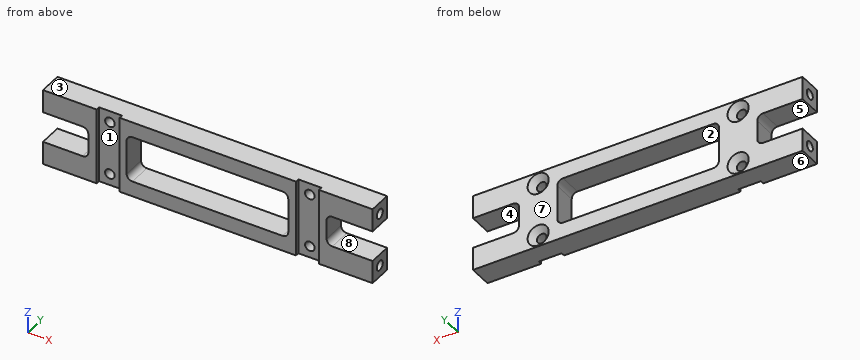
```python
from build123d import *

# Parameters (mm, degrees)
SKETCH2_W                   = 86
SKETCH2_H                   = 20
BOSS_EXTRUDE1_DEPTH         = 6
TAP_DRILL_FOR_M3_TAP2_D     = 2.5
TAP_DRILL_FOR_M3_TAP2_DEPTH = 8
TAP_DRILL_FOR_M3_TAP2_TIP   = 0.751075774
TAP_DRILL_FOR_M3_TAP1_D     = 2.5
TAP_DRILL_FOR_M3_TAP1_DEPTH = 8
TAP_DRILL_FOR_M3_TAP1_TIP   = 0.751075774
SKETCH7_W                   = 6
SKETCH7_H                   = 20
CUT_EXTRUDE1_DEPTH          = 1
TAP_DRILL_FOR_M3X0_5_TAP1_D = 2.5
CHAMFER1_SIZE               = 1.5
CUT_EXTRUDE2_REACH          = 90.499
SKETCH9_W                   = 42.171572875
SKETCH9_H                   = 12
SKETCH9_W_2                 = 11.828427125
SKETCH9_H_2                 = 8
SKETCH9_W_3                 = 12
FILLET1_R                   = 1.5


with BuildPart() as part:
    # Sketch2 → Boss-Extrude1 (new body)
    with BuildSketch(Plane(origin=(0, 0, 0), x_dir=(1, 0, 0), z_dir=(0, 1, 0))):
        with Locations((43, -10)):
            Rectangle(SKETCH2_W, SKETCH2_H)
    extrude(amount=BOSS_EXTRUDE1_DEPTH)

    # Tap Drill for M3 Tap2
    with Locations(Plane(origin=(86, 0.779165189, 7.640466368), x_dir=(0, 0, -1), z_dir=(1, 0, 0))):
        with Locations((-9.359533632, 2.220834811), (4.640466368, 2.220834811)):
            Hole(TAP_DRILL_FOR_M3_TAP2_D / 2, depth=TAP_DRILL_FOR_M3_TAP2_DEPTH)
            with Locations((0, 0, -(TAP_DRILL_FOR_M3_TAP2_DEPTH + TAP_DRILL_FOR_M3_TAP2_TIP / 2))):  # 118° drill point
                Cone(0, TAP_DRILL_FOR_M3_TAP2_D / 2, TAP_DRILL_FOR_M3_TAP2_TIP, mode=Mode.SUBTRACT)

    # Tap Drill for M3 Tap1
    with Locations(Plane.ZY):
        with Locations((3, 3), (17, 3)):
            Hole(TAP_DRILL_FOR_M3_TAP1_D / 2, depth=TAP_DRILL_FOR_M3_TAP1_DEPTH)
            with Locations((0, 0, -(TAP_DRILL_FOR_M3_TAP1_DEPTH + TAP_DRILL_FOR_M3_TAP1_TIP / 2))):  # 118° drill point
                Cone(0, TAP_DRILL_FOR_M3_TAP1_D / 2, TAP_DRILL_FOR_M3_TAP1_TIP, mode=Mode.SUBTRACT)

    # Sketch7 → Cut-Extrude1 (cut)
    with BuildSketch(Plane.XZ):
        with Locations((17, 10)):
            Rectangle(SKETCH7_W, SKETCH7_H)
        with Locations((69, 10)):
            Rectangle(SKETCH7_W, SKETCH7_H)
    extrude(amount=-CUT_EXTRUDE1_DEPTH, mode=Mode.SUBTRACT)

    # Tap Drill for M3x0.5 Tap1 (through all)
    with Locations(Plane(origin=(16.828427125, 1, 17), x_dir=(0, 0, -1), z_dir=(0, -1, 0))):
        with Locations((0, 0), (14, 0), (0, 52.171572875), (14, 52.171572875)):
            Hole(TAP_DRILL_FOR_M3X0_5_TAP1_D / 2)

    # Chamfer1
    chamfer1_edges = [part.edges().sort_by_distance(p)[0] for p in [
        (69, 6, 1.75),
        (69, 6, 15.75),
        (16.828427125, 6, 1.75),
        (16.828427125, 6, 15.75),
    ]]
    chamfer(chamfer1_edges, length=CHAMFER1_SIZE)

    # Sketch9 → Cut-Extrude2 (cut, up to next)
    with BuildSketch(Plane(origin=(0, 6, 0), x_dir=(1, 0, 0), z_dir=(0, 1, 0)), mode=Mode.PRIVATE) as cut_extrude2_sk1:
        with Locations((42.914213563, -10)):
            Rectangle(SKETCH9_W, SKETCH9_H)
    cut_extrude2_tool1 = extrude(cut_extrude2_sk1.sketch, amount=-CUT_EXTRUDE2_REACH, mode=Mode.PRIVATE) & part.part
    # Sketch9 → Cut-Extrude2 (cut, up to next)
    with BuildSketch(Plane(origin=(0, 6, 0), x_dir=(1, 0, 0), z_dir=(0, 1, 0)), mode=Mode.PRIVATE) as cut_extrude2_sk2:
        with Locations((5.914213563, -10)):
            Rectangle(SKETCH9_W_2, SKETCH9_H_2)
    cut_extrude2_tool2 = extrude(cut_extrude2_sk2.sketch, amount=-CUT_EXTRUDE2_REACH, mode=Mode.PRIVATE) & part.part
    # Sketch9 → Cut-Extrude2 (cut, up to next)
    with BuildSketch(Plane(origin=(0, 6, 0), x_dir=(1, 0, 0), z_dir=(0, 1, 0)), mode=Mode.PRIVATE) as cut_extrude2_sk3:
        with Locations((80, -10)):
            Rectangle(SKETCH9_W_3, SKETCH9_H_2)
    cut_extrude2_tool3 = extrude(cut_extrude2_sk3.sketch, amount=-CUT_EXTRUDE2_REACH, mode=Mode.PRIVATE) & part.part
    add(cut_extrude2_tool1.solids().sort_by_distance((42.914214, 6, 10))[0], mode=Mode.SUBTRACT)
    add(cut_extrude2_tool2.solids().sort_by_distance((5.914214, 6, 10))[0], mode=Mode.SUBTRACT)
    add(cut_extrude2_tool3.solids().sort_by_distance((80, 6, 10))[0], mode=Mode.SUBTRACT)

    # Fillet1
    fillet1_edges = [part.edges().sort_by_distance(p)[0] for p in [
        (21.828427125, 3, 16),
        (21.828427125, 3, 4),
        (64, 3, 4),
        (64, 3, 16),
        (11.828427125, 3, 6),
        (11.828427125, 3, 14),
        (74, 3, 14),
        (74, 3, 6),
    ]]
    fillet(fillet1_edges, radius=FILLET1_R)


solid = part.part
```
Can you work these out from the model? Positions are in its coordinate system, mm. Face numbers are marked on the shaded views. A direction names the side the tool comes from. Coordinates: 2 decimals unless noted, no trailing zeros. Write each loop counter-clockwise with the first axis right and the second up, starting at its lowest first coordinate (ties: lowest second). Pieces come first, ordered by that corner, then holes. Notation, with made-up numbers: (48, -33) - (86, -33) arc R22 cw to (86, -2) - close; hole circle Ø7 at (55, 4). An arc over 180 degrees is marked (long way). Return JSON: item names as keys, results as strings.
Q1. I'm going to push flat-ended pins straight in: pin 1 Ø2 at (y, z) = (3, 3) entering from -X; pin 2 Ø1.1 at (y, z) = (0.5, 10.5) entering from -X; pin 3 Ø3 at (x, z) = (70, 12) entering from -Y; pin 4 Ø6.5 at (x, z) = (15.5, 10) entering from -Y. Where does each tip first touch, or does it pass through?
Computed values:
{"pin 1": "stops at x = 8.15", "pin 2": "stops at x = 11.83", "pin 3": "stops at y = 1", "pin 4": "stops at y = 0"}
Q2. If we section it at A-A (x = 58): Please give me the cut outline in (y, z), then the cut area to 3 significant figures.
Computed values:
{"outline": "(0, 0) - (6, 0) - (6, 4) - (0, 4) - close; (0, 16) - (6, 16) - (6, 20) - (0, 20) - close", "area": "48.0 mm2"}
Q3. Please list where these lines run through material, in increasing order: L1, parallel to Z at x = 82.5, y = 3; L2, parallel to X at y = 1.2, z = 3; L3, parallel to Z at x = 69, y = 1.75. Write a range as from..to.
Computed values:
{"L1": "z = 0..1.75, 4.25..6, 14..15.75, 18.25..20", "L2": "x = 0..15.58, 18.08..67.75, 70.25..86", "L3": "z = 0..1.75, 4.25..15.75, 18.25..20"}
Q4. Thinking about a two-plate mould opening in Z: for the marked faces 6, 7 and 8, which applies, +Z half, -Z half, draft (parallel to the pull), parting line (faces both ways), or undercut?
Computed values:
{"face 6": "-Z half", "face 7": "draft", "face 8": "undercut"}
Q5. If we section it at B-B (x = 69): Please give me the cut outline in (y, z), then the cut area to 3 significant figures.
Computed values:
{"outline": "(1, 0) - (6, 0) - (6, 0.25) - (4.5, 1.75) - (1, 1.75) - close; (1, 4.25) - (4.5, 4.25) - (6, 5.75) - (6, 14.25) - (4.5, 15.75) - (1, 15.75) - close; (1, 18.25) - (4.5, 18.25) - (6, 19.75) - (6, 20) - (1, 20) - close", "area": "70.5 mm2"}
Q6. On a 3-axis mill with a long thin cutter (end or side, diameter ignored), from which of +Z, -Z, +X, -X, +Y, -Y can I reach the whole of each face in a straight line? I mean the marked faces 1, 2, 3, 4 and 5. Say none if no direction works.
Computed values:
{"face 1": "+Z, -Z, -Y", "face 2": "+Y, -Y", "face 3": "+Z, +X, -X, +Y, -Y", "face 4": "+X, +Y, -Y", "face 5": "-X, +Y, -Y"}
